Input: part model. Units: mm. Frame: model coordinates. Coordinates: 2 decimals unless noted, no trailing zeros. Loops run counter-clockwise (first coordinate to the right, second up) from the corner with the lowest first, then second, coordinate; pieces in that order, holes last. Notation, with made-up numbers: M 16,9.25 L 64,9.25 A32 ccw 64,40.25 Z; hole C 2.25,80 d2. An arc over 180 degrees is marked long. Use a Markdown table: item, result. Add a question column.
1. Section B-B on y = 74.5. Output: boundary loops of the cut face in (x, z).
2. Pin query (flat end, axial travel): pin 1 (1.5 mm diameter, centred on x = 4, z = 0, fed in from -Y). Return the tip coordinate at first contact, or that it passes through.
3. Section A-A on x = 0.5. State how many separate pieces and enclosed holes the cut face has, then the cut area to 3 significant figures.
4. Line query: L1, parallel to Z at x = 4, y = 61; L2, parallel to X at y = 78, z = 1; L3, parallel to X at y = 61, z = 1. Output: solid intervals per line, ascending. Write a range as [from, to].
```python
from build123d import *

# Parameters (mm, degrees)
SKETCH_1_W                   = 13
SKETCH_1_H                   = 6
EXTRUDE_1_DEPTH              = 100
CUT_EXTRUDE_1_DEPTH          = 101.390487597
CUT_EXTRUDE_1_DEPTH_BACK     = 101.390487597
HOLE_WIZARD_M3_1_D           = 2.5
HOLE_WIZARD_M3_1_CSINK_D     = 3.05
HOLE_WIZARD_M3_1_CSINK_ANGLE = 90


with BuildPart() as part:
    # 草图1 → 凸台-拉伸1 (new body)
    with BuildSketch(Plane(origin=(0, 0, 0), x_dir=(1, 0, 0), z_dir=(0, 1, 0))):
        Rectangle(SKETCH_1_W, SKETCH_1_H)
    extrude(amount=EXTRUDE_1_DEPTH)

    # 草图2 → 切除-拉伸1 (cut, two sides: drawn at the far end of the back side and taken through both)
    with BuildSketch(Plane(origin=(0, 0, -3), x_dir=(-1, 0, 0), z_dir=(0, 0, -1)).offset(-CUT_EXTRUDE_1_DEPTH_BACK)):
        Polygon((-1.732050808, 13), (-3.464101615, 10), (-1.732050808, 7), (1.732050808, 7), (3.464101615, 10), (1.732050808, 13), align=None)
        Polygon((-1.732050808, 23), (-3.464101615, 20), (-1.732050808, 17), (1.732050808, 17), (3.464101615, 20), (1.732050808, 23), align=None)
        Polygon((-1.732050808, 33), (-3.464101615, 30), (-1.732050808, 27), (1.732050808, 27), (3.464101615, 30), (1.732050808, 33), align=None)
        Polygon((-1.732050808, 43), (-3.464101615, 40), (-1.732050808, 37), (1.732050808, 37), (3.464101615, 40), (1.732050808, 43), align=None)
        Polygon((-1.732050808, 53), (-3.464101615, 50), (-1.732050808, 47), (1.732050808, 47), (3.464101615, 50), (1.732050808, 53), align=None)
        Polygon((-1.732050808, 63), (-3.464101615, 60), (-1.732050808, 57), (1.732050808, 57), (3.464101615, 60), (1.732050808, 63), align=None)
        Polygon((-1.732050808, 73), (-3.464101615, 70), (-1.732050808, 67), (1.732050808, 67), (3.464101615, 70), (1.732050808, 73), align=None)
        Polygon((-1.732050808, 83), (-3.464101615, 80), (-1.732050808, 77), (1.732050808, 77), (3.464101615, 80), (1.732050808, 83), align=None)
        Polygon((-1.732050808, 93), (-3.464101615, 90), (-1.732050808, 87), (1.732050808, 87), (3.464101615, 90), (1.732050808, 93), align=None)
    extrude(amount=CUT_EXTRUDE_1_DEPTH + CUT_EXTRUDE_1_DEPTH_BACK, mode=Mode.SUBTRACT)

    # M3 螺纹孔1 (through all)
    with Locations(Plane(origin=(0, 0, 0), x_dir=(-1, 0, 0), z_dir=(0, -1, 0))):
        with Locations((4, 0), (-4, 0)):
            CounterSinkHole(HOLE_WIZARD_M3_1_D / 2, HOLE_WIZARD_M3_1_CSINK_D / 2, counter_sink_angle=HOLE_WIZARD_M3_1_CSINK_ANGLE)


solid = part.part
```
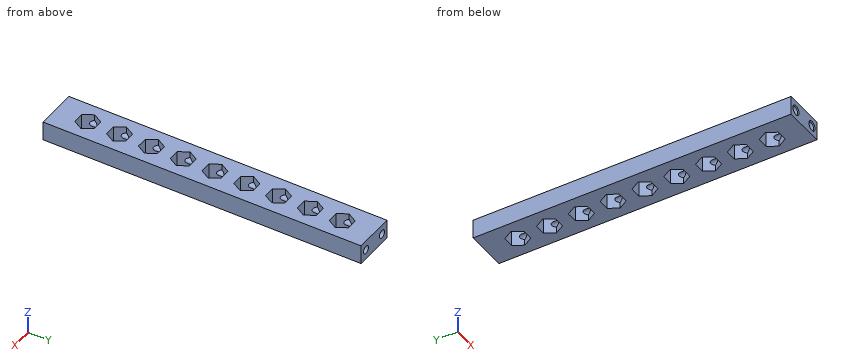
Answers below:
| question | item | result |
|---|---|---|
| 1 | outline | M -6.5,-3 L 6.5,-3 L 6.5,3 L -6.5,3 Z; hole C -4,0 d2.5; hole C 4,0 d2.5 |
| 2 | pin 1 | passes through |
| 3 | separate pieces | 10 |
| 3 | enclosed holes | 0 |
| 3 | area | 276 mm² |
| 4 | L1 | z = [-3, -1.25], [1.25, 3] |
| 4 | L2 | x = [-6.5, -4.75], [-3.25, -2.31], [2.31, 3.25], [4.75, 6.5] |
| 4 | L3 | x = [-6.5, -4.75], [-3.25, -2.89], [2.89, 3.25], [4.75, 6.5] |
